from build123d import *

# Parameters (mm, degrees)
BOSS_EXTRUDE1_DEPTH = 20
SKETCH2_W           = 12.2
SKETCH2_H           = 16
CUT_EXTRUDE1_DEPTH  = 1


with BuildPart() as part:
    # Sketch1 → Boss-Extrude1 (new body)
    with BuildSketch(Plane(origin=(0, 0, 0), x_dir=(1, 0, 0), z_dir=(0, 1, 0))):
        Polygon((69.282032303, 0), (34.641016151, 60), (-34.641016151, 60), (-69.282032303, 0), (-34.641016151, -60), (34.641016151, -60), align=None)
    extrude(amount=BOSS_EXTRUDE1_DEPTH)

    # Sketch2 → Cut-Extrude1 (cut)
    with BuildSketch(Plane(origin=(0, 20, 0), x_dir=(1, 0, 0), z_dir=(0, 1, 0))):
        with Locations((-18.541016151, 52)):
            Rectangle(SKETCH2_W, SKETCH2_H)
        with Locations((18.541016151, 52)):
            Rectangle(SKETCH2_W, SKETCH2_H)
        Polygon((64.282032303, -8.660254038), (50.425625842, -0.660254038), (44.325625842, -11.225763964), (58.182032303, -19.225763964), align=None)
        Polygon((45.741016151, -40.774236036), (31.884609691, -32.774236036), (25.784609691, -43.339745962), (39.641016151, -51.339745962), align=None)
        Polygon((-39.641016151, -51.339745962), (-25.784609691, -43.339745962), (-31.884609691, -32.774236036), (-45.741016151, -40.774236036), align=None)
        Polygon((-58.182032303, -19.225763964), (-44.325625842, -11.225763964), (-50.425625842, -0.660254038), (-64.282032303, -8.660254038), align=None)
    extrude(amount=-CUT_EXTRUDE1_DEPTH, mode=Mode.SUBTRACT)


solid = part.part
Source: CAD feature listing. Evaluate the final solid. Frame: model axes, mm. A direction names the side the tool comes from. Give positions to 0.01 mm unless a question says otherwise; leave off trailing zeros. Write each loop counter-clockwise with the first axis right and the second up, starting at its lowest first coordinate (ties: lowest second). Pieces come first, ordered by that corner, then holes. Notation, with made-up numbers: M -12,71 L 20,71 A23 cw 20,97 Z; hole C 32.25,0.5 d11. An arc over 180 degrees is marked long. Return JSON: item names as keys, results as strings. Group by question number.
1) Draft query along X for faces 1 (the face through (0, 10, 60)), 2 (the face through (-57.257, 19.507, 4.604)), 3 (the face through (-51.72, 9.86, -30.42)). Return one class per face: released by +X, released by -X, zero draft, split by the parting line, or undercut.
2) Cut plane C-C, the plane x = 54.5. Output: boundary loops of the cut face in (y, z).
3) Ray query, L1, parallel to X at y = 11.5, z = 32; L2, parallel to X at y = 11, z = -11; L3, parallel to Z at x = -57, y = 14.25. Return the intervals inside material, ascending.
4) Cut plane A-A, the plane y = 14.5. Output: boundary loops of the cut face in (x, z), then the cut area to 3 significant figures.
5) First-contact query: pin 1 Ø4 at (x, y) = (47, 4) entering from +Z; pin 2 Ø4 at (x, z) = (-55, -29.5) entering from -Y; pin 3 Ø4 at (x, y) = (-42, 6) entering from +Z; pin 4 Ø0.8 at (x, y) = (-20.5, 19.5) entering from -Z. Flat tips, straight axial feed; report the tip coordinate or a pass-through.
6) Set-up query: faces 4 (the face through (18, 19, -52)), 5 (the face through (-32.81, 19.507, 47.396)), 6 (the face through (-1, 0, -1)), 7 (the face through (-1, 20, -1)), 8 (the face through (-47.33, 19.51, 6.02)). Return all of +Z, -Z, +X, -X, +Y, -Y with unobstructed straight access to the full face (end or side cutting, diameter ignored); none if empty.
7) Cut plane B-B, the plane z = 45.5. Output: boundary loops of the cut face in (x, y), then the cut area to 3 significant figures.
8) Cut plane D-D, the plane z = -49. Output: boundary loops of the cut face in (x, y).
Data:
{
 "1": {"face 1": "zero draft", "face 2": "undercut", "face 3": "released by -X"},
 "2": {"outline": "M 0,-25.6 L 20,-25.6 L 20,3.01 L 19,3.01 L 19,17.1 L 20,17.1 L 20,25.6 L 0,25.6 Z"},
 "3": {"L1": "x = -50.81 to 50.81", "L2": "x = -62.93 to 62.93", "L3": "z = -21.27 to 21.27"},
 "4": {"outline": "M -69.28,0 L -34.64,-60 L 34.64,-60 L 69.28,0 L 34.64,60 L -34.64,60 Z", "area": "12,500 mm²"},
 "5": {"pin 1": "stops at z = 42.06", "pin 2": "passes through", "pin 3": "stops at z = 50.72", "pin 4": "stops at z = -44"},
 "6": {"face 4": "-Z, +Y", "face 5": "-X, +Y", "face 6": "+Z, -Z, +X, -X, -Y", "face 7": "+Z, -Z, +X, -X, +Y", "face 8": "+Y"},
 "7": {"outline": "M -43.01,0 L 43.01,0 L 43.01,19 L 29.53,19 L 29.53,20 L -29.53,20 L -29.53,19 L -43.01,19 Z", "area": "1,690 mm²"},
 "8": {"outline": "M -40.99,0 L 40.99,0 L 40.99,20 L 24.64,20 L 24.64,19 L 12.44,19 L 12.44,20 L -12.44,20 L -12.44,19 L -24.64,19 L -24.64,20 L -40.99,20 Z"}
}
